```python
from build123d import *

# Parameters (mm, degrees)
F1_DEPTH  = 8
F3_T      = -1.5
F2_R      = 1.5
F4_DEPTH  = 196
F6_DEPTH  = 196.001
F7_R      = 3
F9_DEPTH  = 196.001
F11_DEPTH = 196.001


with BuildPart() as f1:
    # F0 (on Top) → F1 (new body)
    with BuildSketch(Plane.XY):
        with BuildLine():
            Line((145.992111, 12.24232), (-50.007889, 12.24232))
            Line((-50.007889, 12.24232), (-50.007889, -2.75768))
            ThreePointArc((-50.007889, -2.75768), (-40.007889, -12.75768), (-50.007889, -22.75768))
            Line((-50.007889, -22.75768), (-50.007889, -37.75768))
            Line((-50.007889, -37.75768), (145.992111, -37.75768))
            Line((145.992111, -37.75768), (145.992111, -22.75768))
            ThreePointArc((145.992111, -22.75768), (135.992111, -12.75768), (145.992111, -2.75768))
            Line((145.992111, -2.75768), (145.992111, 12.24232))
        make_face()
    extrude(amount=F1_DEPTH)

    # F3
    f3_openings = [f1.faces().sort_by_distance(p)[0] for p in [
        (47.992111, -12.75768, 0),
    ]]
    offset(amount=F3_T, openings=f3_openings)

    # F2 (on face) → F4 (join, through all)
    with BuildSketch(Plane.YZ.offset(145.992111)):
        with Locations((7.24232, 2)):
            Circle(F2_R)
        with Locations((-32.75768, 2)):
            Circle(F2_R)
    extrude(amount=-F4_DEPTH)

    # F5 (on face) → F6 (cut, through all)
    with BuildSketch(Plane(origin=(-50.007889, 0, 0), x_dir=(0, -1, 0), z_dir=(-1, 0, 0))):
        with BuildLine():
            ThreePointArc((-15.24232, 1.255437), (-17.447156, 3.75963), (-18.24232, 7))
            Line((-18.24232, 7), (-18.24232, 0.071797))
            ThreePointArc((-18.24232, 0.071797), (-16.673224, 0.488491), (-15.24232, 1.255437))
        make_face()
        with BuildLine():
            ThreePointArc((-12.24232, 7), (-13.037483, 3.75963), (-15.24232, 1.255437))
            ThreePointArc((-15.24232, 1.255437), (-13.811415, 0.488491), (-12.24232, 0.071797))
            Line((-12.24232, 0.071797), (-12.24232, 7))
        make_face()
        with BuildLine():
            ThreePointArc((-12.24232, 0.071797), (-13.811415, 0.488491), (-15.24232, 1.255437))
            ThreePointArc((-15.24232, 1.255437), (-16.673224, 0.488491), (-18.24232, 0.071797))
            Line((-18.24232, 0.071797), (-18.24232, 0))
            Line((-18.24232, 0), (-12.24232, 0))
            Line((-12.24232, 0), (-12.24232, 0.071797))
        make_face()
        with BuildLine():
            Line((-18.24232, 0), (-18.24232, 0.071797))
            ThreePointArc((-18.24232, 0.071797), (-18.741033, 0.017972), (-19.24232, 0))
            Line((-19.24232, 0), (-18.24232, 0))
        make_face()
        with BuildLine():
            ThreePointArc((-11.24232, 0), (-11.743607, 0.017972), (-12.24232, 0.071797))
            Line((-12.24232, 0.071797), (-12.24232, 0))
            Line((-12.24232, 0), (-11.24232, 0))
        make_face()
    extrude(amount=-F6_DEPTH, mode=Mode.SUBTRACT)

    # F7
    f7_edges = [f1.edges().sort_by_distance(p)[0] for p in [
        (47.992111, -37.75768, 8),
        (47.992111, 12.24232, 8),
        (145.992111, 4.74232, 8),
        (145.992111, -30.25768, 8),
        (135.992111, -12.75768, 8),
        (-50.007889, 4.74232, 8),
        (-40.007889, -12.75768, 8),
        (-50.007889, -30.25768, 8),
        (145.992111, -37.75768, 4),
        (145.992111, 12.24232, 4.035898),
        (-50.007889, -37.75768, 4),
        (145.992111, -2.75768, 4),
        (145.992111, -22.75768, 4),
    ]]
    fillet(f7_edges, radius=F7_R)

    # F8 (on face) → F9 (cut, through all)
    with BuildSketch(Plane.YZ.offset(145.992111)):
        with BuildLine():
            ThreePointArc((-17.512412, 5), (-21.047946, 3.535534), (-22.512412, 0))
            Line((-22.512412, 0), (-3.16584, 0))
            ThreePointArc((-3.16584, 0), (-4.630306, 3.535534), (-8.16584, 5))
            Line((-8.16584, 5), (-17.512412, 5))
        make_face()
    extrude(amount=-F9_DEPTH, mode=Mode.SUBTRACT)

    # F10 (on face) → F11 (cut, through all)
    with BuildSketch(Plane.YZ.offset(145.992111)):
        with BuildLine():
            ThreePointArc((-32.75768, 0), (-33.779229, 0.105468), (-34.75768, 0.417424))
            Line((-34.75768, 0.417424), (-34.75768, 5))
            Line((-34.75768, 5), (-37.75768, 5))
            Line((-37.75768, 5), (-37.75768, 0))
            Line((-37.75768, 0), (-32.75768, 0))
        make_face()
        with BuildLine():
            Line((7.24232, 0), (7.751559, 0))
            Line((7.751559, 0), (12.24232, 0))
            Line((12.24232, 0), (12.24232, 5))
            Line((12.24232, 5), (9.238324, 5))
            Line((9.238324, 5), (9.238324, 0.415683))
            ThreePointArc((9.238324, 0.415683), (8.261734, 0.105024), (7.24232, 0))
        make_face()
    extrude(amount=-F11_DEPTH, mode=Mode.SUBTRACT)


solid = f1.part
```
Source: CAD feature listing. Evaluate the final solid. Frame: model axes, mm. A direction names the side the tool comes from. Coordinates: 2 decimals unless noted, no trailing zeros. Write each loop counter-clockwise with the first axis right and the second up, starting at its lowest first coordinate (ties: lowest second). Pieces come first, ordered by that corner, then holes. Notation, with made-up numbers: (43.5, 3.5) -> (62.5, 3.5) arc R19 ccw to (62.5, 25.5) -> close; hole circle Ø11 at (84.5, 65.5). An arc over 180 degrees is marked (long way). Return JSON: item names as keys, results as strings. Group by question number.
1) Section query B-B, the plane y = -27.5. Return loops of the section in (x, z), plus the area to 3 significant figures.
2) Ray query, line 1 along X through (y, z) = (-30, 0.5); line 2 along Z through (x, y) = (22.5, -15.5); line 3 along X through (y, z) = (-30.5, 6.25). Return the intervals inside material, ascending.
3) Mould query, pull axis Z, two halves, no side actions, for faces 4 (the face through (145.992, -30, 2)), 5 (the face through (144.492, 3, 3)), 6 (the face through (-48.508, 3, 3)), 7 (the face through (-49, 1, 0)). Classes: +Z half, -Z half, draft (parallel to the pull), parting line (faces both ways), or undercut.
4) Contact query for flat-ended pins moving along their axis: P1, Ø1.2, axis at x = 145.5, z = 3, coming from the -Y side; P2, Ø1.5, axis at x = 83.5, y = 11.5, coming from the -Z side; P3, Ø4, axis at x = 99.5, y = 4, coming from the -Z side. Output: stop coordinate, or through.
5) Section query A-A, the plane x = 16. Return loops of the section in (y, z), plus the area to 3 significant figures.
6) Set-up query: faces 1 (the face through (-43.65, -21.6, 2.88)), 2 (the face through (144.492, -29, 3)), 3 (the face through (141.71, -3.72, 3.23)). Return all of +Z, -Z, +X, -X, +Y, -Y with unobstructed straight access to the full face (end or side cutting, diameter ignored); none if empty.
From the geometry:
{
 "1": {"outline": "(-50.01, 0) -> (-48.51, 0) -> (-48.51, 6.5) -> (144.49, 6.5) -> (144.49, 0) -> (145.99, 0) -> (145.99, 5) arc R3 ccw to (142.99, 8) -> (-47.01, 8) arc R3 ccw to (-50.01, 5) -> close", "area": "310 mm²"},
 "2": {"line 1": "-50.01 to -48.51, 144.49 to 145.99", "line 2": "6.5 to 8", "line 3": "-49.74 to -48.51, 144.49 to 145.72"},
 "3": {"face 4": "draft", "face 5": "undercut", "face 6": "undercut", "face 7": "-Z half"},
 "4": {"P1": "y = -34.76", "P2": "z = 5", "P3": "z = 1.16"},
 "5": {"outline": "(-37.76, 5) -> (-36.26, 5) -> (-36.26, 6.5) -> (10.74, 6.5) -> (10.74, 5) -> (12.24, 5) arc R3 ccw to (9.24, 8) -> (-34.76, 8) arc R3 ccw to start; circle Ø3 at (-32.76, 2); circle Ø3 at (7.24, 2)", "area": "89.8 mm²"},
 "6": {"face 1": "-Z, +X, -X", "face 2": "none", "face 3": "+Z, -Z, +X"}
}
